Could you check a few things on this model? Use its own coordinates, in mm. A direction names the side the tool comes from. Round coordinates to 2 decimals unless told otherwise and drop trailing zeros. Write each loop counter-clockwise with the first axis right and the second up, starting at its lowest first coordinate (ties: lowest second). Pieces come first, ordered by that corner, then holes. Notation, with made-up numbers: (-26, 88) -> (27, 88) arc R23 ccw to (27, 126) -> close; hole circle Ø7 at (-14, 81.5). An arc over 180 degrees is marked (long way). Answer in a Markdown table with one row per item. Add a question column.
```python
from build123d import *

# Parameters (mm, degrees)
SKETCH_1_R      = 11
EXTRUDE_1_DEPTH = 20
SKETCH_2_R      = 13.5
EXTRUDE_2_DEPTH = 15
FILLET_1_R      = 5


with BuildPart() as part:
    # 草图1 → 凸台-拉伸1 (new body)
    with BuildSketch(Plane.XY):
        with Locations((-173.275516994, 0)):
            Circle(SKETCH_1_R)
    extrude(amount=EXTRUDE_1_DEPTH)

    # 草图2 → 凸台-拉伸2 (add)
    with BuildSketch(Plane.XY.offset(20)):
        with Locations((-173.275516994, 0)):
            Circle(SKETCH_2_R)
    extrude(amount=EXTRUDE_2_DEPTH)

    # 圆角1
    fillet_1_edges = [part.edges().sort_by_distance(p)[0] for p in [
        (-186.775516994, 0, 35),
    ]]
    fillet(fillet_1_edges, radius=FILLET_1_R)


solid = part.part
```
(1) Suppose I cut it at B-B, the plane z = 25. Please give me the cut outline in (x, y), then the cut area to 3 significant figures.
(2) For P1, Ø8, axis at x = -173, z = 11, coming from the -Y side; P2, Ø4, axis at y = 1.5, z = 11, coming from the +X side; P3, Ø1.5, axis at x = -162.5, z = 18.5, coming from the +Y side, each with a flat end and sliding along its axis, tell me the tip position at first contact or that it passes through.
(3) I need wall thicknesses on L1, parallel to X at y = -0.25, z = 5; L2, parallel to Y at x = -181, z = 31; L3, parallel to X at y = -11.25, z = 31. Which ranges of each line are inside material? Lowest first, please.
(4) Suppose I cut it at C-C, the plane z = 12. Please give me the cut outline in (x, y).
(5) Suppose I cut it at A-A, the plane y = 0. Please give me the cut outline in (x, z).
(6) On a 3-axis mill with a long thin cutter (end or side, diameter ignored), from which of +Z, -Z, +X, -X, +Y, -Y can I reach the whole of each face in a straight line? I mean faces 1 (the face through (-160.805, -5.171, 24.93)), 2 (the face through (-162.783, 3.304, 9.86)). Say none if no direction works.
Response:
| question | item | result |
|---|---|---|
| 1 | outline | circle Ø27 at (-173.28, 0) |
| 1 | area | 573 mm² |
| 2 | P1 | y = -11 |
| 2 | P2 | x = -162.28 |
| 2 | P3 | y = 4.53 |
| 3 | L1 | -184.27 to -162.28 |
| 3 | L2 | -10.95 to 10.95 |
| 3 | L3 | -180.55 to -166 |
| 4 | outline | circle Ø22 at (-173.28, 0) |
| 5 | outline | (-186.78, 20) -> (-184.28, 20) -> (-184.28, 0) -> (-162.28, 0) -> (-162.28, 20) -> (-159.78, 20) -> (-159.78, 30) arc R5 ccw to (-164.78, 35) -> (-181.78, 35) arc R5 ccw to (-186.78, 30) -> close |
| 6 | face 1 | +Z, -Z |
| 6 | face 2 | -Z |
